Source: CAD feature listing. Evaluate the final solid. Frame: model axes, mm. Give positions to 0.01 mm unless a question says otherwise; leave off trailing zeros. Write each loop counter-clockwise with the first axis right and the second up, starting at its lowest first coordinate (ties: lowest second). Pieces come first, ordered by that corner, then holes. Notation, with made-up numbers: (10.25, 86) -> (51.25, 86) arc R9 cw to (51.25, 98) -> close; hole circle Ø3 at (5, -2). An arc over 180 degrees is marked (long way). Write item = value, one per line.
Autodesk Inventor part; units mm, degrees
ref_plane "YZ Plane" through (0, 0, 0) normal (1, 0, 0) x (0, 1, 0)
ref_plane "XZ Plane" through (0, 0, 0) normal (0, 1, 0) x (-1, 0, 0)
ref_plane "XY Plane" through (0, 0, 0) normal (0, 0, 1) x (1, 0, 0)
sketch "Sketch1" plane through (0, 0, 0) normal (0, 1, 0) x (-1, 0, 0)
  circle A0 centre (0, 0) radius 9 construction
  circle A1 centre (0, 0) radius 7 construction
  circle A2 centre (12, -12) radius 1.715
  line L0 (0, 0) -> (0, -7) construction
  line L1 (0, 0) -> (9, 0) construction
  circle A3 centre (0, 0) radius 3.175
  line L2 (18, -66) -> (-138, -66)
  line L3 (-138, -66) -> (-138, 18)
  line L4 (-138, 18) -> (18, 18)
  line L5 (18, 18) -> (18, -66)
  circle A4 centre (12, 12) radius 1.715
  circle A5 centre (-12, 12) radius 1.715
  circle A6 centre (-12, -12) radius 1.715
  line L6 (12, -12) -> (0, 0) construction
  circle A7 centre (0, -24) radius 3.175
  circle A8 centre (12, -36) radius 1.715
  circle A9 centre (-12, -36) radius 1.715
  circle A10 centre (0, -48) radius 3.175
  circle A11 centre (12, -60) radius 1.715
  circle A12 centre (-12, -60) radius 1.715
  circle A13 centre (-36, 12) radius 1.715
  circle A14 centre (-24, 0) radius 3.175
  circle A15 centre (-36, -12) radius 1.715
  circle A16 centre (-24, -24) radius 3.175
  circle A17 centre (-36, -36) radius 1.715
  circle A18 centre (-24, -48) radius 3.175
  circle A19 centre (-36, -60) radius 1.715
  circle A20 centre (-60, 12) radius 1.715
  circle A21 centre (-48, 0) radius 3.175
  circle A22 centre (-60, -12) radius 1.715
  circle A23 centre (-48, -24) radius 3.175
  circle A24 centre (-60, -36) radius 1.715
  circle A25 centre (-48, -48) radius 3.175
  circle A26 centre (-60, -60) radius 1.715
  circle A27 centre (-84, 12) radius 1.715
  circle A28 centre (-72, 0) radius 3.175
  circle A29 centre (-84, -12) radius 1.715
  circle A30 centre (-72, -24) radius 3.175
  circle A31 centre (-84, -36) radius 1.715
  circle A32 centre (-72, -48) radius 3.175
  circle A33 centre (-84, -60) radius 1.715
  circle A34 centre (-108, 12) radius 1.715
  circle A35 centre (-96, 0) radius 3.175
  circle A36 centre (-108, -12) radius 1.715
  circle A37 centre (-96, -24) radius 3.175
  circle A38 centre (-108, -36) radius 1.715
  circle A39 centre (-96, -48) radius 3.175
  circle A40 centre (-108, -60) radius 1.715
  circle A41 centre (-132, 12) radius 1.715
  circle A42 centre (-120, 0) radius 3.175
  circle A43 centre (-132, -12) radius 1.715
  circle A44 centre (-120, -24) radius 3.175
  circle A45 centre (-132, -36) radius 1.715
  circle A46 centre (-120, -48) radius 3.175
  circle A47 centre (-132, -60) radius 1.715
  dimension "d0" = 18
  dimension "d1" = 2
  dimension "d2" = 3.43
  dimension "d6" = 6.35
  dimension "d27" = 360
  dimension "d29" = 45
  dimension "d30" = 12
  dimension "d33" = 24
  dimension "d40" = 24
  dimension "d45" = 6
  dimension "d46" = 6
  dimension "d47" = 6
  dimension "d48" = 6
extrude "Extrusion3" add sketch "Sketch1" along normal blind 5.95
equation "\"d0\" = 0.75 * BearingDiameter"
equation "\"d1\" = SiliconeOverlapThickness"
equation "\"d2\" = HoldScrewDiameter"
equation "\"d6\" = DowlDiameter"
equation "\"d49\" = WoodThickness"
equation "\"BearingDiameter\" = 24"
properties part number "BearingSiliconeMold_1" material "MDF Medium Density Fiberboard"
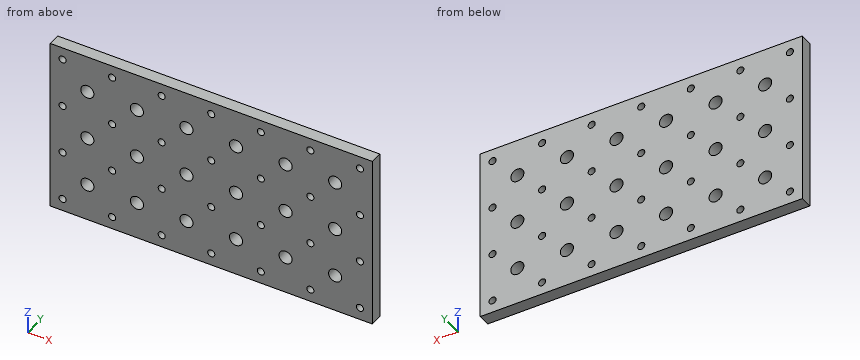
1) Material intervals for L1, parallel to Z at x = 84, y = 2.85 (3 decimals); L2, parallel to Z at x = 48, y = 1.7 (3 decimals); L3, parallel to Z at x = 45.5, y = 2.75, sorted ascending.
Computed:
L1 = -66 to -61.715, -58.285 to -37.715, -34.285 to -13.715, -10.285 to 10.285, 13.715 to 18
L2 = -66 to -51.175, -44.825 to -27.175, -20.825 to -3.175, 3.175 to 18
L3 = -66 to -49.96, -46.04 to -25.96, -22.04 to -1.96, 1.96 to 18
2) Cut plane C-C (x = 48). Return the cut outline in (y, z) (3 decimals).
Computed:
outline = (0, -66) -> (5.95, -66) -> (5.95, -51.175) -> (0, -51.175) -> close; (0, -44.825) -> (5.95, -44.825) -> (5.95, -27.175) -> (0, -27.175) -> close; (0, -20.825) -> (5.95, -20.825) -> (5.95, -3.175) -> (0, -3.175) -> close; (0, 3.175) -> (5.95, 3.175) -> (5.95, 18) -> (0, 18) -> close
3) Contact query for a flat-ended pin moving along its axis: pin 1 (3 mm diameter, centred on x = 84, z = -60, fed in from +Y). Output: stop coordinate, or through.
Computed:
pin_1 = through
4) Cut plane A-A (z = 12). State how many separate pieces and enclosed holes the cut face has, then the cut area to 3 significant figures.
Computed:
separate_pieces = 8
enclosed_holes = 0
area = 785 mm²
5) Cut plane B-B (x = -12). Return the cut outline in (y, z) (3 decimals).
Computed:
outline = (0, -66) -> (5.95, -66) -> (5.95, -61.715) -> (0, -61.715) -> close; (0, -58.285) -> (5.95, -58.285) -> (5.95, -37.715) -> (0, -37.715) -> close; (0, -34.285) -> (5.95, -34.285) -> (5.95, -13.715) -> (0, -13.715) -> close; (0, -10.285) -> (5.95, -10.285) -> (5.95, 10.285) -> (0, 10.285) -> close; (0, 13.715) -> (5.95, 13.715) -> (5.95, 18) -> (0, 18) -> close
